from build123d import *

# Parameters (mm, degrees)
SKETCH1_R           = 25
BOSS_EXTRUDE1_DEPTH = 5
SKETCH3_R           = 25
SKETCH3_R_2         = 22
BOSS_EXTRUDE3_DEPTH = 10
SKETCH4_R           = 9
BOSS_EXTRUDE4_DEPTH = 14
SKETCH5_R           = 2.5
CUT_EXTRUDE1_DEPTH  = 15
SKETCH6_W           = 5.5
SKETCH6_H           = 3
CUT_EXTRUDE2_DEPTH  = 6
CUT_EXTRUDE3_START  = 1.83304
SKETCH7_R           = 1.7
CUT_EXTRUDE3_DEPTH  = 7.16696
CUT_EXTRUDE4_DEPTH  = 15.0000001
CIRPATTERN1_COUNT   = 6
CHAMFER1_SIZE       = 0.25


with BuildPart() as part:
    # Sketch1 → Boss-Extrude1 (new body)
    with BuildSketch(Plane.XY):
        Circle(SKETCH1_R)
    extrude(amount=BOSS_EXTRUDE1_DEPTH)

    # Sketch3 → Boss-Extrude3 (add)
    with BuildSketch(Plane.XY):
        Circle(SKETCH3_R)
        Circle(SKETCH3_R_2, mode=Mode.SUBTRACT)
    extrude(amount=BOSS_EXTRUDE3_DEPTH)

    # Sketch4 → Boss-Extrude4 (add)
    with BuildSketch(Plane.XY):
        Circle(SKETCH4_R)
    extrude(amount=BOSS_EXTRUDE4_DEPTH)

    # Sketch5 → Cut-Extrude1 (cut, through all)
    with BuildSketch(Plane.XY):
        Circle(SKETCH5_R)
    extrude(amount=CUT_EXTRUDE1_DEPTH, mode=Mode.SUBTRACT)

    # Sketch6 → Cut-Extrude2 (cut)
    with BuildSketch(Plane.XY.offset(14)):
        with Locations((0, 4.75)):
            Rectangle(SKETCH6_W, SKETCH6_H)
    extrude(amount=-CUT_EXTRUDE2_DEPTH, mode=Mode.SUBTRACT)

    # Sketch7 → Cut-Extrude3 (cut)
    with BuildSketch(Plane(origin=(0, 0, 0), x_dir=(1, 0, 0), z_dir=(0, 1, 0)).offset(CUT_EXTRUDE3_START)):
        with Locations((0, -11)):
            Circle(SKETCH7_R)
    extrude(amount=CUT_EXTRUDE3_DEPTH, mode=Mode.SUBTRACT)

    # Sketch8 → Cut-Extrude4 (cut, through all)
    with BuildSketch(Plane.XY):
        with BuildLine():
            Line((-4.392304845, 16.392304845), (-3.614211274, 13.488420103))
            ThreePointArc((-3.614211274, 13.488420103), (-3.178915308, 12.899635496), (-2.459122201, 12.765293494))
            ThreePointArc((-2.459122201, 12.765293494), (0, 13), (2.459122201, 12.765293494))
            ThreePointArc((2.459122201, 12.765293494), (3.178915308, 12.899635496), (3.614211274, 13.488420103))
            Line((3.614211274, 13.488420103), (4.392304845, 16.392304845))
            ThreePointArc((4.392304845, 16.392304845), (4.277317186, 17.176389762), (3.627930726, 17.630601766))
            ThreePointArc((3.627930726, 17.630601766), (0, 18), (-3.627930726, 17.630601766))
            ThreePointArc((-3.627930726, 17.630601766), (-4.277317186, 17.176389762), (-4.392304845, 16.392304845))
        make_face()
    cut_extrude4 = extrude(amount=CUT_EXTRUDE4_DEPTH, mode=Mode.SUBTRACT)

    # CirPattern1: Cut-Extrude4 ×6 about axis
    cirpattern1_axis = Axis((0, 0, 0), (0, 0, 1))
    for i in range(1, CIRPATTERN1_COUNT):
        add(cut_extrude4.rotate(cirpattern1_axis, i * 360 / CIRPATTERN1_COUNT), mode=Mode.SUBTRACT)

    # Chamfer1
    chamfer1_edges = [part.edges().sort_by_distance(p)[0] for p in [
        (-25, 0, 0),
        (-25, 0, 10),
    ]]
    chamfer(chamfer1_edges, length=CHAMFER1_SIZE)


solid = part.part
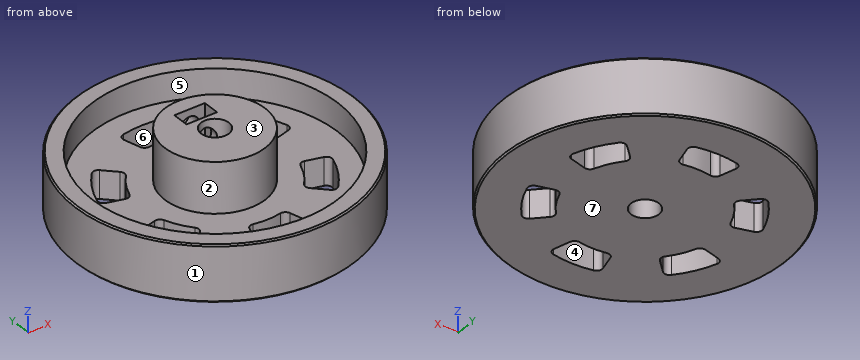
Geometry: final body of the model. Coordinates: model frame, mm. Face numbers are marked on the shaded views. A direction names the side the tool comes from. Give positions to 0.01 mm unless a question says otherwise; leave off trailing zeros. Write each loop counter-clockwise with the first axis right and the second up, starting at its lowest first coordinate (ties: lowest second). Pieces come first, ordered by that corner, then holes. Notation, with made-up numbers: M 12.5,1 L 45.5,1 A22 ccw 45.5,13 Z; hole C 16,-1.5 d9. An arc over 180 degrees is marked long. Answer in a Markdown table with one row per item. Add a question column.
(1) First-contact query: pin 1 (2 mm diameter, centred on x = -16, y = -18.5, fed in from +Z); pin 2 (1.6 mm diameter, centred on x = 0, z = 11, fed in from +Y); pin 3 (2 mm diameter, centred on y = 5.5, z = 4.5, fed in from -X). Flat tips, straight axial feed; report the tip coordinate or a pass-through.
(2) Section A-A on y = 0. Return loops of the section in (x, z).
(3) Ray query, line 1 (Y direction, x = 0, z = 7.5); line 2 (X direction, y = 10, z = 1); line 3 (Z direction, x = -11, y = -12). Return the intervals inside material, ascending.
(4) Section C-C on x = 0. State how many separate pieces and enclosed holes the cut face has, and give its area (3 significant figures).
(5) Mould query, pull axis X, two halves, no side actions, for the marked faces 1, 2, 3 and 4. Classes: +X half, -X half, draft (parallel to the pull), parting line (faces both ways), or undercut.
(6) Section B-B on z = 6.5. Return loops of the section in (x, y), and give its area (3 significant figures).
(7) Reachability of the marked faces 5, 6 and 7 from +Z, -Z, +X, -X, +Y, -Y: full face, straight path, thin tool, end or side. Return the list, or none.
Result set:
| question | item | result |
|---|---|---|
| 1 | pin 1 | stops at z = 10 |
| 1 | pin 2 | stops at y = -2.37 |
| 1 | pin 3 | stops at x = -24.59 |
| 2 | outline | M -25,0.25 L -24.75,0 L -2.5,0 L -2.5,14 L -9,14 L -9,5 L -22,5 L -22,10 L -24.75,10 L -25,9.75 Z; M 2.5,0 L 24.75,0 L 25,0.25 L 25,9.75 L 24.75,10 L 22,10 L 22,5 L 9,5 L 9,14 L 2.5,14 Z |
| 3 | line 1 | y = -25 to -22, -9 to -2.5, 2.5 to 9, 22 to 25 |
| 3 | line 2 | x = -22.91 to -14.97, -10 to 10, 14.97 to 22.91 |
| 3 | line 3 | z = 0 to 5 |
| 4 | separate pieces | 6 |
| 4 | enclosed holes | 0 |
| 4 | area | 292 mm^2 |
| 5 | face 1 | parting line |
| 5 | face 2 | undercut |
| 5 | face 3 | draft |
| 5 | face 4 | undercut |
| 6 | outline | C 0,0 d50; C 0,0 d18; hole C 0,0 d44; hole C 0,0 d5 |
| 6 | area | 678 mm^2 |
| 7 | face 5 | +Z |
| 7 | face 6 | +Z, -Z |
| 7 | face 7 | -Z, +X, -X, +Y, -Y |
